Autodesk Inventor part; units mm, degrees
ref_plane "YZ Plane" through (0, 0, 0) normal (1, 0, 0) x (0, 1, 0)
ref_plane "XZ Plane" through (0, 0, 0) normal (0, 1, 0) x (-1, 0, 0)
ref_plane "XY Plane" through (0, 0, 0) normal (0, 0, 1) x (1, 0, 0)
sketch "スケッチ1" plane through (0, 0, 0) normal (0, 0, 1) x (1, 0, 0)
  circle A0 centre (-18.2979, -11.3675) radius 1.05 construction
  circle A1 centre (-0.7979, 13.5) radius 1.05 construction
  circle A2 centre (12.2021, -13.5) radius 1.05 construction
  circle A3 centre (-18.2979, 10.6325) radius 1.05 construction
  circle A4 centre (-10.7975, 0) radius 1.3 construction
  circle A5 centre (-9.5382, 13.5) radius 1.05
  circle A6 centre (-9.5382, -13.5) radius 1.05
  circle A7 centre (17.4618, 13.5) radius 1.05
  circle A8 centre (17.4618, -13.5) radius 1.05
  line L0 (-11.7979, -16) -> (18.2021, -16)
  arc A9 (18.2021, -16) -> (20.2021, -14) centre (18.2021, -14) ccw
  line L1 (20.2021, -14) -> (20.2021, 14)
  arc A10 (20.2021, 14) -> (18.2021, 16) centre (18.2021, 14) ccw
  line L2 (18.2021, 16) -> (-11.7979, 16)
  line L3 (-22.7979, 0) -> (0, 0) construction
  line L4 (0, 0) -> (13.5202, -23.4176) construction
  line L5 (-22.7979, 0) -> (-32.6431, 0) construction
  line L6 (9.2376, -16) -> (3.5384, -19.2904) construction
  line L7 (11.7376, -20.3301) -> (14.3357, -18.8301) construction
  line L8 (9.2376, 16) -> (3.5384, 19.2904) construction
  line L9 (11.7376, 20.3301) -> (14.3357, 18.8301) construction
  circle A11 centre (17.4618, -13.5) radius 2.5 construction
  circle A12 centre (17.4618, 13.5) radius 2.5 construction
  line L10 (3.6668, -16) -> (18.2021, -16)
  arc A13 (18.2021, -16) -> (20.2021, -14) centre (18.2021, -14) ccw
  line L11 (3.6668, 16) -> (18.2021, 16)
  arc A14 (20.2021, 14) -> (18.2021, 16) centre (18.2021, 14) ccw
  line L12 (-5.7966, 16) -> (-11.7979, 16)
  arc A15 (-11.7979, 16) -> (-13.3279, 15.9267) centre (-11.7979, 0) ccw
  line L13 (-5.7966, -16) -> (-11.7979, -16)
  arc A16 (-13.3279, -15.9267) -> (-11.7979, -16) centre (-11.7979, 0) ccw
  arc A17 (-13.5809, -10.642) -> (-13.5809, 10.642) centre (-10.7975, 0) ccw
  line L14 (-13.3279, -15.9267) -> (-13.5809, -10.642)
  line L15 (-13.5809, 10.642) -> (-13.3279, 15.9267)
  line L16 (20.2021, 0) -> (35.2021, 0) construction
  line L17 (20.2021, -22.5) -> (20.2021, -17.0694)
  line L18 (20.2021, -9.9306) -> (20.2021, 9.9306)
  line L19 (20.2021, 0) -> (35.2021, 0)
  line L20 (20.2021, -17.0694) -> (20.2021, -14)
  line L21 (17.4618, 17) -> (35.2021, 17)
  line L22 (20.2021, 14) -> (20.2021, -28)
  line L23 (20.2021, 17) -> (65.2021, 17) construction
  line L24 (20.2021, -28) -> (35.2021, -28)
  line L25 (35.2021, -28) -> (35.2021, 17)
  line L26 (27.7021, -28) -> (27.7021, 17) construction
  line L27 (27.7021, -5.5) -> (20.2021, -5.5) construction
  circle A18 centre (27.7021, -17.5) radius 1.6
  circle A19 centre (27.7021, 6.5) radius 1.6
  line L28 (17.4618, 13.5) -> (17.4618, 14.55)
  line L29 (17.4618, 16) -> (17.4618, 17)
  point P0 (-22.7979, -6.4363)
  point P1 (15.7302, -16)
  point P2 (13.5202, 23.4176)
  point P3 (15.7302, 16)
  dimension "d0" = 120
  dimension "d7" = 5
  dimension "d10" = 5
  dimension "d24" = 22
  dimension "d28" = 15
  dimension "d38" = 3.5
  dimension "d39" = 45
  dimension "d40" = 90
  dimension "d41" = 15
  dimension "d42" = 2.7403
  dimension "d43" = 3.2
  dimension "d44" = 12
extrude "押し出し5" add sketch "スケッチ1" along normal blind 3
properties part number "デュアルサーボつなぎフレーム_アルミ(A2017)_t1.5" material "アルミニウム 6061"
The listing builds one solid part. Answer for the finished solid, in the listing's coordinates (mm). Give positions to 0.01 mm unless a question says otherwise; leave off trailing zeros. Order: outer loops, then holes, each group sorted by start corner. A loop starts at its lowest first (then second) coordinate and runs counter-clockwise, first axis right, second up. Notation, with made-up numbers: (23, -23.75) - (28, -23.75) arc R28 ccw to (28, 8.25) - close; hole circle Ø10 at (-18, -15.5). An arc over 180 degrees is marked (long way). Use one line per item in the form item = value.
1) Each of these flat-tipped pins is pushed along its axis until it touches: pin 1 (2.5 mm diameter, centred on x = -9.54, y = -13.5, fed in from -Z); pin 2 (1.5 mm diameter, centred on x = 13, z = 1.5, fed in from -Y); pin 3 (1.5 mm diameter, centred on x = 8, z = 2, fed in from +Y). Where does it stop, or does it pass through?
Verdict:
pin_1 = 0
pin_2 = -16
pin_3 = 16
2) Consider probe 1 along Y at (x, z) = (-1, 2.25); probe 2 along Y at (x, z) = (3.5, 0.6); probe 3 along Y at (x, z) = (-3.5, 1). Determine where each line is inside the solid, lowest interval first. Write a range as [from, to].
Verdict:
probe_1 = [-16, -5], [5, 16]
probe_2 = [-16, 16]
probe_3 = [-16, -8.23], [8.23, 16]
3) Find section A-A on z = 1.7. Determine the outline of the cut face in (x, y), and give its area (3 significant figures).
Verdict:
outline = (-13.58, -10.64) - (-13.33, -15.93) arc R15.99 ccw to (-11.8, -16) - (18.2, -16) arc R2 ccw to (20.2, -14) - (20.2, -28) - (35.2, -28) - (35.2, 17) - (17.46, 17) - (17.46, 16) - (-11.8, 16) arc R16.01 ccw to (-13.33, 15.93) - (-13.58, 10.64) arc R11 cw (long way) to start; hole circle Ø2.1 at (-9.54, -13.5); hole circle Ø2.1 at (-9.54, 13.5); hole circle Ø2.1 at (17.46, -13.5); hole circle Ø2.1 at (17.46, 13.5); hole circle Ø3.2 at (27.7, -17.5); hole circle Ø3.2 at (27.7, 6.5)
area = 1,480 mm^2
4) Find section D-D on x = 4.5. Determine the outline of the cut face in (y, z).
Verdict:
outline = (-16, 0) - (16, 0) - (16, 3) - (-16, 3) - close
5) Find section C-C on x = -6.5. Determine the outline of the cut face in (y, z).
Verdict:
outline = (-16, 0) - (-10.13, 0) - (-10.13, 3) - (-16, 3) - close; (10.13, 0) - (16, 0) - (16, 3) - (10.13, 3) - close
6) The mould has two halves that part along Y. Classify faces 1 (the flat face through (35.202, -6, 1)), 2 (the flat face through (3, 16, 1)), 3 (the cylindrical face through (18, 12.6, 1.5)), 4 (the cylindrical face through (0.2, 0.3, 1.5)): released by +Y, released by -Y, zero draft, split by the parting line, or undercut.
Verdict:
face_1 = zero draft
face_2 = released by +Y
face_3 = undercut
face_4 = undercut
7) Find section B-B on y = -17.5. Determine the outline of the cut face in (x, z), and give its area (3 significant figures).
Verdict:
outline = (20.2, 0) - (26.1, 0) - (26.1, 3) - (20.2, 3) - close; (29.3, 0) - (35.2, 0) - (35.2, 3) - (29.3, 3) - close
area = 35.4 mm^2
